Build history of the part. All positions in model axes, mm. A direction names the side the tool comes from. Round coordinates to 2 decimals unless told otherwise and drop trailing zeros. Write each loop counter-clockwise with the first axis right and the second up, starting at its lowest first coordinate (ties: lowest second). Pieces come first, ordered by that corner, then holes. Notation, with made-up numbers: (-16, 55.25) -> (1, 55.25) arc R25 cw to (1, 76.25) -> close; hole circle Ø1 at (43.25, 7). An arc over 180 degrees is marked (long way). Answer in a Markdown table with one row per item. Add a question column.
Autodesk Inventor part; units mm, degrees
ref_plane "YZ Plane" through (0, 0, 0) normal (1, 0, 0) x (0, 1, 0)
ref_plane "XZ Plane" through (0, 0, 0) normal (0, 1, 0) x (-1, 0, 0)
ref_plane "XY Plane" through (0, 0, 0) normal (0, 0, 1) x (1, 0, 0)
sketch "Boceto1" plane through (0, 0, 0) normal (0, 0, 1) x (1, 0, 0)
  line L0 (0, 0) -> (100, 0)
  line L1 (100, 0) -> (100, 100)
  line L2 (100, 100) -> (0, 100)
  line L3 (0, 100) -> (0, 0)
  line L4 (0, 100) -> (5, 100)
  circle A0 centre (5, 95) radius 4
  line L5 (0, 0) -> (0, 5)
  circle A1 centre (5, 5) radius 4
  line L6 (100, 0) -> (100, 5)
  circle A2 centre (95, 5) radius 4
  line L7 (100, 100) -> (95, 100)
  circle A3 centre (95, 95) radius 4
  line L8 (0, 100) -> (50, 100)
  line L9 (50, 100) -> (50, 50)
  dimension "d6" = 100
  dimension "d7" = 100
  dimension "d10" = 8
  dimension "d20" = 50
  dimension "d21" = 50
extrude "Extrusión1" add sketch "Boceto1" along normal blind 50
fillet "Empalme1" radius 1 4 edges at (100, 0, 25) (0, 0, 25) (100, 100, 25) (0, 100, 25)
sketch "Boceto2" plane through (0, 0, 50) normal (0, 0, 1) x (1, 0, 0)
  circle A0 centre (50, 50) radius 25
  point P0 (0, 0)
  dimension "d27" = 50
extrude "Extrusión2" add sketch "Boceto2" along normal blind 50
sketch "Boceto3" plane through (50, 50, 100) normal (0, 0, 1) x (1, 0, 0)
  circle A0 centre (0, 0) radius 20
  point P0 (-50, -50)
  dimension "d30" = 40
extrude "Extrusión3" cut sketch "Boceto3" against normal blind 30
thread "Rosca1"
properties part number "Tarea 1 Joel Monroy Lab Din"
(1) Saw through at A-A (y = 5). List the corners of the cut face in (x, z), plus the area to 3 significant figures.
(2) Mould opens along Y. For faces 1 (the face through (6.846, 98.549, 24.65)), 2 (the face through (27, 62, 50)), 3 (the face through (69.076, 56.007, 85.21)), 4 (the face through (51, 100, 25)) say: pulls with the +Y half, pulls with the -Y half, needs draft (parallel to the pull), parting line crosses it, or undercut.
(3) Probe line 1 along Y through (x, z) = (95, 19); line 2 along Z through (x, y) = (39.5, 41); line 3 along Z through (x, y) = (29, 95). List the from-to ranges inside material, lowest first.
(4) Drop flat-ended pins along their axis: P1, Ø5, axis at x = 12.5, y = 58, coming from the +Z side; P2, Ø24, axis at x = 50, y = 50, coming from the +Z side; P3, Ø2, axis at y = 70, z = 86.5, coming from the -X side. Give the stop position or say it passes through.
(5) Saw through at D-D (y = 50). List the corners of the cut face in (x, z).
(6) Which spindle directions (+Z, -Z, +X, -X, +Y, -Y) get a long thin tool onto all of the face, cutting with end or side? Do faces 5 (the face through (30, 65, 75)), 6 (the face through (91, 5, 25)). Say none if no direction does.
(7) Saw through at C-C (z = 33). List the corners of the cut face in (x, y), plus the area to 3 significant figures.
Answer sheet:
| question | item | result |
|---|---|---|
| 1 | outline | (0, 0) -> (1, 0) -> (1, 50) -> (0, 50) -> close; (9, 0) -> (91, 0) -> (91, 50) -> (9, 50) -> close; (99, 0) -> (100, 0) -> (100, 50) -> (99, 50) -> close |
| 1 | area | 4,200 mm² |
| 2 | face 1 | undercut |
| 2 | face 2 | needs draft |
| 2 | face 3 | undercut |
| 2 | face 4 | pulls with the +Y half |
| 3 | line 1 | y = 0 to 1, 9 to 91, 99 to 100 |
| 3 | line 2 | z = 0 to 70 |
| 3 | line 3 | z = 0 to 50 |
| 4 | P1 | stops at z = 50 |
| 4 | P2 | stops at z = 70 |
| 4 | P3 | stops at x = 33.75 |
| 5 | outline | (0, 0) -> (100, 0) -> (100, 50) -> (75, 50) -> (75, 100) -> (70, 100) -> (70, 70) -> (30, 70) -> (30, 100) -> (25, 100) -> (25, 50) -> (0, 50) -> close |
| 6 | face 5 | +Z |
| 6 | face 6 | +Z, -Z |
| 7 | outline | (0, 1) arc R1 ccw to (1, 0) -> (99, 0) arc R1 ccw to (100, 1) -> (100, 99) arc R1 ccw to (99, 100) -> (1, 100) arc R1 ccw to (0, 99) -> close; hole circle Ø8 at (5, 5); hole circle Ø8 at (5, 95); hole circle Ø8 at (95, 5); hole circle Ø8 at (95, 95) |
| 7 | area | 9,800 mm² |
